Source: CAD feature listing. Evaluate the final solid. Frame: model axes, mm. A direction names the side the tool comes from. Give positions to 0.01 mm unless a question says otherwise; leave off trailing zeros. Write each loop counter-clockwise with the first axis right and the second up, starting at its lowest first coordinate (ties: lowest second). Pieces come first, ordered by that corner, then holes. Notation, with made-up numbers: M -9.5,-20 L 40.5,-20 A26 cw 40.5,16 Z; hole C 55,52.25 d1. An arc over 180 degrees is marked long. Return JSON: item names as keys, results as strings.
```python
from build123d import *

# Parameters (mm, degrees)
SKETCH1_W           = 205.763637231
SKETCH1_H           = 129.455055738
BOSS_EXTRUDE1_DEPTH = 889.508
SKETCH2_W           = 34.228088198
SKETCH2_H           = 27.935874949
CUT_EXTRUDE1_DEPTH  = 1151.636
SKETCH3_W           = 34.228088198
SKETCH3_H           = 27.935874949
CUT_EXTRUDE2_DEPTH  = 1331.214
FILLET3_R           = 25.4
FILLET4_R           = 25.4
FILLET5_R           = 25.4
FILLET7_R           = 25.4
SKETCH4_W           = 12.650207524
SKETCH4_H           = 27.935874949
BOSS_EXTRUDE3_DEPTH = 874.268
SKETCH5_W           = 12.621373824
SKETCH5_H           = 27.935874949
CUT_EXTRUDE5_DEPTH  = 1063.752
SKETCH6_W           = 12.913753515
SKETCH6_H           = 27.935874949
CUT_EXTRUDE6_DEPTH  = 1244.346
SKETCH8_W           = 46.849462022
SKETCH8_H           = 50.759590395
CUT_EXTRUDE7_DEPTH  = 508
SKETCH9_W           = 47.141841713
SKETCH9_H           = 50.759590395
CUT_EXTRUDE8_DEPTH  = 508
SKETCH10_R          = 7.658892277
CUT_EXTRUDE9_DEPTH  = 263.652


with BuildPart() as part:
    # Sketch1 → Boss-Extrude1 (new body)
    with BuildSketch(Plane(origin=(0, 0, 0), x_dir=(1, 0, 0), z_dir=(0, 1, 0))):
        with Locations((102.881818616, -64.727527869)):
            Rectangle(SKETCH1_W, SKETCH1_H)
    extrude(amount=BOSS_EXTRUDE1_DEPTH)

    # Sketch2 → Cut-Extrude1 (cut)
    with BuildSketch(Plane(origin=(0, 889.508, 0), x_dir=(1, 0, 0), z_dir=(0, 1, 0))):
        with Locations((17.114044099, -64.727527869)):
            Rectangle(SKETCH2_W, SKETCH2_H)
    extrude(amount=-CUT_EXTRUDE1_DEPTH, mode=Mode.SUBTRACT)

    # Sketch3 → Cut-Extrude2 (cut)
    with BuildSketch(Plane(origin=(0, 889.508, 0), x_dir=(1, 0, 0), z_dir=(0, 1, 0))):
        with Locations((188.649593132, -64.727527869)):
            Rectangle(SKETCH3_W, SKETCH3_H)
    extrude(amount=-CUT_EXTRUDE2_DEPTH, mode=Mode.SUBTRACT)

    # Fillet3
    fillet3_edges = [part.edges().sort_by_distance(p)[0] for p in [
        (0, 444.754, 0),
    ]]
    fillet(fillet3_edges, radius=FILLET3_R)

    # Fillet4
    fillet4_edges = [part.edges().sort_by_distance(p)[0] for p in [
        (205.763637231, 444.754, 0),
    ]]
    fillet(fillet4_edges, radius=FILLET4_R)

    # Fillet5
    # the kernel refuses this fillet: 25.4 mm, written as the material it takes off along each edge
    with BuildSketch(Plane(origin=(205.763637231, 953.008, 50.759590394), x_dir=(0, 0, -1), z_dir=(0, -1, 0))) as fillet5_piece_1:
        with BuildLine():
            CenterArc((FILLET5_R, -FILLET5_R), FILLET5_R, 90, 90)
            Line((0, -FILLET5_R), (0, 0))
            Line((0, 0), (FILLET5_R, 0))
        make_face()
    extrude(amount=1016.508, mode=Mode.SUBTRACT)

    # Fillet7
    # the kernel refuses this fillet: 25.4 mm, written as the material it takes off along each edge
    with BuildSketch(Plane(origin=(0, 953.008, 50.759590394), x_dir=(0, 0, -1), z_dir=(0, -1, 0))) as fillet7_piece_1:
        with BuildLine():
            CenterArc((FILLET7_R, FILLET7_R), FILLET7_R, 180, 90)
            Line((0, FILLET7_R), (0, 0))
            Line((0, 0), (FILLET7_R, 0))
        make_face()
    extrude(amount=1016.508, mode=Mode.SUBTRACT)

    # Sketch4 → Boss-Extrude3 (add)
    with BuildSketch(Plane(origin=(0, 889.508, 0), x_dir=(1, 0, 0), z_dir=(0, 1, 0))):
        with Locations((40.55319196, -64.727527869)):
            Rectangle(SKETCH4_W, SKETCH4_H)
    extrude(amount=-BOSS_EXTRUDE3_DEPTH)

    # Sketch5 → Cut-Extrude5 (cut)
    with BuildSketch(Plane(origin=(0, 889.508, 0), x_dir=(1, 0, 0), z_dir=(0, 1, 0))):
        with Locations((40.53877511, -64.727527869)):
            Rectangle(SKETCH5_W, SKETCH5_H)
    extrude(amount=-CUT_EXTRUDE5_DEPTH, mode=Mode.SUBTRACT)

    # Sketch6 → Cut-Extrude6 (cut)
    with BuildSketch(Plane(origin=(0, 889.508, 0), x_dir=(1, 0, 0), z_dir=(0, 1, 0))):
        with Locations((165.078672276, -64.727527869)):
            Rectangle(SKETCH6_W, SKETCH6_H)
    extrude(amount=-CUT_EXTRUDE6_DEPTH, mode=Mode.SUBTRACT)

    # Sketch8 → Cut-Extrude7 (cut)
    with BuildSketch(Plane(origin=(0, 889.508, 0), x_dir=(1, 0, 0), z_dir=(0, 1, 0))):
        with Locations((23.424731011, -104.075260541)):
            Rectangle(SKETCH8_W, SKETCH8_H)
    extrude(amount=-CUT_EXTRUDE7_DEPTH, mode=Mode.SUBTRACT)

    # Sketch9 → Cut-Extrude8 (cut)
    with BuildSketch(Plane(origin=(0, 889.508, 0), x_dir=(1, 0, 0), z_dir=(0, 1, 0))):
        with Locations((182.192716375, -104.075260541)):
            Rectangle(SKETCH9_W, SKETCH9_H)
    extrude(amount=-CUT_EXTRUDE8_DEPTH, mode=Mode.SUBTRACT)

    # Sketch10 → Cut-Extrude9 (cut)
    with BuildSketch(Plane.ZY.offset(-46.849462022)):
        with Locations((109.367874663, 857.026947913)):
            Circle(SKETCH10_R)
    extrude(amount=-CUT_EXTRUDE9_DEPTH, mode=Mode.SUBTRACT)


solid = part.part
```
1) Cut plane C-C, the plane y = 693. Return the cut outline in (x, z).
Numbers:
{"outline": "M 0,25.38 A25.4 ccw 25.4,0 L 180.36,0 A25.4 ccw 205.76,25.4 A25.4 ccw 180.36,50.76 L 158.62,50.76 L 158.62,129.46 L 46.85,129.46 L 46.85,50.76 L 25.4,50.76 A25.4 ccw Z"}
2) Set-up query: faces 1 (the face through (36, 451, 50.76)), 2 (the face through (182, 381.508, 104)), 3 (the face through (101, 340, 129.455)), 4 (the face through (101, 889.508, 49)), 5 (the face through (182, 193, 78.695)). Return all of +Z, -Z, +X, -X, +Y, -Y with unobstructed straight access to the full face (end or side cutting, diameter ignored); none if empty.
Numbers:
{"face 1": "-X, +Y, -Y", "face 2": "+Z, +X, +Y", "face 3": "+Z, +X, -X, +Y, -Y", "face 4": "+Z, -Z, +X, -X, +Y", "face 5": "+X, +Y, -Y"}
3) Line query: line 1 (X direction, y = 852.5, z = 86); line 2 (Z direction, x = 183, y = 203); line 3 (Y direction, x = 46.5, z = 106.5). Output: solid intervals per line, ascending. Write a range as [from, to].
Numbers:
{"line 1": "x = [46.85, 158.62]", "line 2": "z = [0.14, 50.62], [78.7, 129.46]", "line 3": "y = [0, 381.51]"}
4) Cut plane B-B, the plane z = 70.5. Return the cut outline in (x, y).
Numbers:
{"outline": "M 46.85,0 L 158.62,0 L 158.62,889.51 L 46.85,889.51 Z"}
5) Draft query along Z for faces 6 (the face through (23, 381.508, 104)), 7 (the face through (23, 193, 78.695)), 8 (the face through (102, 439, 0)). Return one class per face: released by +Z, released by -Z, zero draft, split by the parting line, or undercut.
Numbers:
{"face 6": "zero draft", "face 7": "undercut", "face 8": "released by -Z"}
6) Contact query for flat-ended pins moving along their axis: pin 1 Ø8 at (y, z) = (447, 62.5) entering from +X; pin 2 Ø6.5 at (x, y) = (40, 504.5) entering from +Z; pin 3 Ø14 at (y, z) = (857.03, 109.37) entering from +X. Output: stop coordinate, or through.
Numbers:
{"pin 1": "stops at x = 158.62", "pin 2": "stops at z = 50.76", "pin 3": "passes through"}
7) Cut plane A-A, the plane y = 271. Return the cut outline in (x, z).
Numbers:
{"outline": "M 0,25.38 A25.4 ccw 25.4,0 L 180.36,0 A25.4 ccw 205.76,25.4 A25.4 ccw 180.36,50.76 L 158.62,50.76 L 158.62,78.7 L 205.76,78.7 L 205.76,129.46 L 0,129.46 L 0,78.7 L 46.85,78.7 L 46.85,50.76 L 25.4,50.76 A25.4 ccw Z"}
